from build123d import *

# Parameters (mm, degrees)
F0_R     = 3
F1_DEPTH = 3
F2_R     = 5
F3_DEPTH = 8
F4_R     = 2
F5_DEPTH = 2
F6_R     = 1.99999
F7_R     = 2.5
F8_DEPTH = 8


# Not quite as in the source:
# - a fillet or chamfer is up to 0.001 mm smaller than in the source, because OpenCascade refuses the exact size


with BuildPart() as f1:
    # F0 (on Top) → F1 (new body)
    with BuildSketch(Plane.XY):
        Circle(F0_R)
    extrude(amount=F1_DEPTH)

    # F2 (on face) → F3 (join)
    with BuildSketch(Plane.XY.offset(3)):
        Circle(F2_R)
    extrude(amount=F3_DEPTH)

    # F4 (on face) → F5 (join)
    with BuildSketch(Plane.XY.offset(11)):
        Circle(F4_R)
    extrude(amount=F5_DEPTH)

    # F6 (radius 2 in the source; OpenCascade refuses exactly that, so slightly less here)
    f6_edges = [f1.edges().sort_by_distance(p)[0] for p in [
        (-5, 0, 11),
        (-5, 0, 3),
    ]]
    fillet(f6_edges, radius=F6_R)

    # F7 (on face) → F8 (cut)
    with BuildSketch(Plane(origin=(0, 0, 0), x_dir=(1, 0, 0), z_dir=(0, 0, -1))):
        Circle(F7_R)
    extrude(amount=-F8_DEPTH, mode=Mode.SUBTRACT)


solid = f1.part
Can you work these out from the model? Positions are in its coordinate system, mm. A direction names the side the tool comes from. Coordinates: 2 decimals unless noted, no trailing zeros. Write each loop counter-clockwise with the first axis right and the second up, starting at its lowest first coordinate (ties: lowest second). Pieces come first, ordered by that corner, then holes. Notation, with made-up numbers: M -6.5,34 L 17.5,34 A18 ccw 17.5,52 Z; hole C 49.25,28.5 d11. An arc over 180 degrees is marked long. Use one line per item in the form item = value.
Q1. For faces 4 (the cylindrical face through (-0.54, 2.44, 3.94)), 5 (the flat face through (-2, 2, 0)), which set-ups out of +Z, -Z, +X, -X, +Y, -Y let a thin tool reach every point of the face, with its end or its side?
Model answer:
face_4 = -Z
face_5 = -Z, +X, -X, +Y, -Y
Q2. For P1, Ø6, axis at x = 0, y = 0, coming from the -Z side; P2, Ø1.5, axis at x = 1.5, y = 0, coming from the -Z side; P3, Ø6, axis at x = -2, z = 11.5, coming from the -Y side; P4, Ø3, axis at x = -4, z = 11, coming from the +Y side, each with a flat end and sliding along its axis, tell me the tip position at first contact or that it passes through.
Model answer:
P1 = 0
P2 = 8
P3 = -4.99
P4 = 3.75
Q3. I need wall thicknesses on line 1 along Y through (x, z) = (0, 6.25); line 2 along Y through (x, z) = (0, 2.5); line 3 along Z through (x, y) = (-1.25, -2). Which ranges of each line are inside material? Lowest first, please. Write a range as from..to.
Model answer:
line_1 = -5..-2.5, 2.5..5
line_2 = -3..-2.5, 2.5..3
line_3 = 8..11
Q4. If we section it at D-D (z = 2.75): Write out the boundary of the cut face in (x, y).
Model answer:
outline = C 0,0 d6; hole C 0,0 d5
Q5. We'd pull the mould along X, two halves only. Please class faces 1 (the cylindrical face through (0, -2, 12)), 2 (the flat face through (1, -2, 11)), 3 (the flat face through (0, 0, 8)): +X half, -X half, draft (parallel to the pull), parting line (faces both ways), or undercut.
Model answer:
face_1 = parting line
face_2 = draft
face_3 = undercut
Q6. If we section it at C-C (z = 5.25): Write out the boundary of the cut face in (x, y), then the cut area to 3 significant figures.
Model answer:
outline = C 0,0 d10; hole C 0,0 d5
area = 58.9 mm^2
